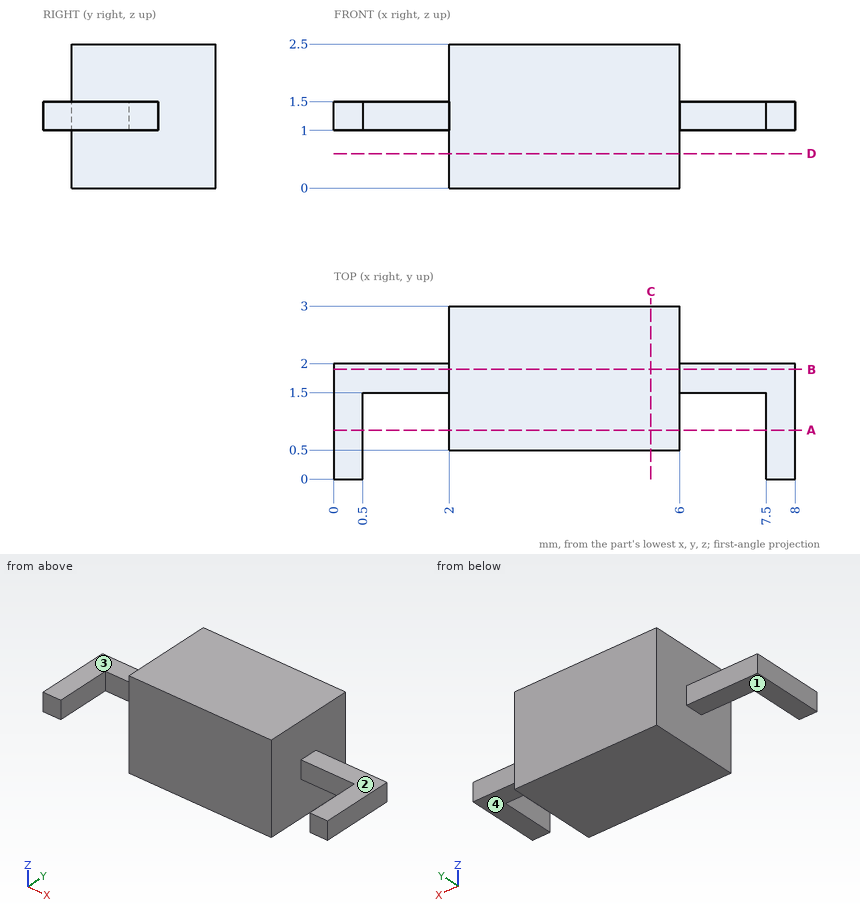
Job drawing, mm, ordinate dimensions from the low corner. One solid piece. A direction names the side the tool comes from. Give positions to 0.01 mm unless a question says otherwise; leave off trailing zeros. Loops run counter-clockwise (first coordinate to the right, second up) from the corner with the lowest first, then second, coordinate; pieces in that order, holes last. Notation, with made-up numbers: (49, 31.5) -> (88, 31.5) arc R7 ccw to (88, 43.5) -> close; hole circle Ø2 at (-31, 8). An arc over 180 degrees is marked (long way). Write each question's results on one line, items separated by ' | '. Start each with the question number.
Q1. Band-saw the part on A-A on y = 0.85. List the corners of the cut face in (x, z), plus the area to 3 significant figures.
Q2. Pin check, flat tips, straight feed: P1, Ø1.6, axis at x = 7, y = 1, coming from the -Z side; P2, Ø0.6, axis at x = 1, y = 1, coming from the +Z side. Stop position of each tip, or through.
Q3. Band-saw the part on D-D on z = 0.6. List the corners of the cut face in (x, y), plus the area to 3 significant figures.
Q4. Band-saw the part on B-B on y = 1.9. List the corners of the cut face in (x, z), plus the area to 3 significant figures.
Q5. Wall check: L1, parallel to Z at x = 7.75, y = 0.2; L2, parallel to X at y = 1.7, z = 1.75; L3, parallel to Y at x = 2.5, z = 0.8. Give the ranges that are in metal, low to high.
Q6. Band-saw the part on C-C on x = 5.5. List the corners of the cut face in (y, z).
Q7. Which spindle directions (+Z, -Z, +X, -X, +Y, -Y) get a long thin tool onto all of the face, cutting with end or side? Do the marked faces 1, 2, 3 and 4. Say none if no direction does.
Results are:
1) outline: (0, 1) -> (0.5, 1) -> (0.5, 1.5) -> (0, 1.5) -> close; (2, 0) -> (6, 0) -> (6, 2.5) -> (2, 2.5) -> close; (7.5, 1) -> (8, 1) -> (8, 1.5) -> (7.5, 1.5) -> close | area: 10.5 mm²
2) P1: stops at z = 1 | P2: passes through
3) outline: (2, 0.5) -> (6, 0.5) -> (6, 3) -> (2, 3) -> close | area: 10.0 mm²
4) outline: (0, 1) -> (2, 1) -> (2, 0) -> (6, 0) -> (6, 1) -> (8, 1) -> (8, 1.5) -> (6, 1.5) -> (6, 2.5) -> (2, 2.5) -> (2, 1.5) -> (0, 1.5) -> close | area: 12.0 mm²
5) L1: z = 1 to 1.5 | L2: x = 2 to 6 | L3: y = 0.5 to 3
6) outline: (0.5, 0) -> (3, 0) -> (3, 2.5) -> (0.5, 2.5) -> close
7) face 1: -Z, -X, +Y, -Y | face 2: +Z, +X, +Y, -Y | face 3: +Z, -X, +Y, -Y | face 4: -Z, +X, +Y, -Y
